Model file for the job. Use its own axes, mm. A direction names the side the tool comes from. Give positions to 0.01 mm unless a question says otherwise; leave off trailing zeros. Write each loop counter-clockwise with the first axis right and the second up, starting at its lowest first coordinate (ties: lowest second). Pieces come first, ordered by that corner, then holes. Notation, with made-up numbers: (-36.75, -16) - (2.25, -16) arc R28 cw to (2.25, 4) - close; hole circle Ø1 at (31, -0.75). An arc over 180 degrees is marked (long way). One line per item, written item: value. Start each with the question number.
(1) Probe L1, parallel to X at y = 0, z = 4.5; L2, parallel to Y at x = 0, z = 7; L3, parallel to Y at x = 0, z = 29.75. List the from-to ranges inside material, lowest first.
(2) Cut at B-B, the plane z = 26.5. List the corners of the cut face in (x, y).
(3) Drop a flat-ended pin along its axis: P1, Ø1, axis at x = 3, y = -1, coming from the -Z side. Give the stop position or say it passes through.
(4) Cut at A-A, the plane z = 8.5. List the corners of the cut face in (x, y), and give its area (3 significant figures).
(5) 3-axis set-ups, long thin cutter, end or side, ignore diameter. For faces 4 (the face through (4, 0, 40)), 5 (the face through (3.233, -1.341, 32.605)), 6 (the face through (-0.867, -3.905, 7.605)): which of +Z, -Z, +X, -X, +Y, -Y reach the whole face in a straight line?
(6) Mould opens along X. For faces 1 (the face through (4.31, -2.535, 19.72)), 2 (the face through (-4.31, 2.535, 19.72)), 3 (the face through (0.151, -0.678, 16.986)) say: pulls with the +X half, pulls with the -X half, needs draft (parallel to the pull), parting line crosses it, or undercut.
from build123d import *

# Parameters (mm, degrees)
BOSS_EXTRUDE1_DEPTH          = 40
SKETCH2_R                    = 3.5
CUT_EXTRUDE1_DEPTH           = 15
F_8_0_8_DIAMETER_HOLE1_D     = 8
F_8_0_8_DIAMETER_HOLE1_DEPTH = 15
F_8_0_8_DIAMETER_HOLE1_TIP   = 2.403442476


with BuildPart() as part:
    # Sketch1 → Boss-Extrude1 (new body)
    with BuildSketch(Plane.XY):
        Polygon((5.773502692, 0), (2.886751346, 5), (-2.886751346, 5), (-5.773502692, 0), (-2.886751346, -5), (2.886751346, -5), align=None)
    extrude(amount=BOSS_EXTRUDE1_DEPTH)

    # Sketch2 → Cut-Extrude1 (cut)
    with BuildSketch(Plane.XY.offset(40)):
        Circle(SKETCH2_R)
    extrude(amount=-CUT_EXTRUDE1_DEPTH, mode=Mode.SUBTRACT)

    # Ø8.0 (8) Diameter Hole1
    with Locations(Plane(origin=(0, 0, 0), x_dir=(-1, 0, 0), z_dir=(0, 0, -1))):
        with Locations((0, 0)):
            Hole(F_8_0_8_DIAMETER_HOLE1_D / 2, depth=F_8_0_8_DIAMETER_HOLE1_DEPTH)
            with Locations((0, 0, -(F_8_0_8_DIAMETER_HOLE1_DEPTH + F_8_0_8_DIAMETER_HOLE1_TIP / 2))):  # 118° drill point
                Cone(0, F_8_0_8_DIAMETER_HOLE1_D / 2, F_8_0_8_DIAMETER_HOLE1_TIP, mode=Mode.SUBTRACT)


solid = part.part
Answers follow:
1. L1: x = -5.77 to -4, 4 to 5.77
1. L2: y = -5 to -4, 4 to 5
1. L3: y = -5 to -3.5, 3.5 to 5
2. outline: (-5.77, 0) - (-2.89, -5) - (2.89, -5) - (5.77, 0) - (2.89, 5) - (-2.89, 5) - close; hole circle Ø7 at (0, 0)
3. P1: stops at z = 15.2
4. outline: (-5.77, 0) - (-2.89, -5) - (2.89, -5) - (5.77, 0) - (2.89, 5) - (-2.89, 5) - close; hole circle Ø8 at (0, 0)
4. area: 36.3 mm²
5. face 4: +Z, +X, -X, +Y, -Y
5. face 5: +Z
5. face 6: -Z
6. face 1: pulls with the +X half
6. face 2: pulls with the -X half
6. face 3: undercut
